from build123d import *

# Parameters (mm, degrees)
BOSS_EXTRUDE1_DEPTH            = 1.93
BOSS_EXTRUDE2_START            = 1.93
BOSS_EXTRUDE2_DEPTH            = 5
BOSS_EXTRUDE3_DEPTH            = 19
CUT_EXTRUDE1_REACH             = 69.337
CUT_EXTRUDE1_DIRECTION_2_REACH = 69.337
FILLET1_R                      = 6
CUT_EXTRUDE2_REACH             = 69.337
SKETCH5_R                      = 3
CUT_EXTRUDE2_DIRECTION_2_REACH = 69.337


with BuildPart() as part:
    # Sketch1 → Boss-Extrude1 (new body)
    # profile 1 of 4: a face of its own
    with BuildSketch(Plane.XY):
        with BuildLine():
            ThreePointArc((32, 27.202941017), (0, 42), (-32, 27.202941017))
            Line((-32, 27.202941017), (-32, 17.202941017))
            Line((-32, 17.202941017), (-37, 11.488655303))
            Line((-37, 11.488655303), (-37, -25.449961479))
            Line((-37, -25.449961479), (-34, -25.449961479))
            Line((-34, -25.449961479), (-34, -26.449961479))
            Line((-34, -26.449961479), (-28, -26.449961479))
            ThreePointArc((-28, -26.449961479), (0, -38.517534478), (28, -26.449961479))
            Line((28, -26.449961479), (34, -26.449961479))
            Line((34, -26.449961479), (34, -25.449961479))
            Line((34, -25.449961479), (37, -25.449961479))
            Line((37, -25.449961479), (37, 11.488655303))
            Line((37, 11.488655303), (32, 17.202941017))
            Line((32, 17.202941017), (32, 27.202941017))
        make_face()
        with BuildLine():
            Line((-13.076696831, -27), (-14, -27))
            ThreePointArc((-14, -27), (-18.345139389, -25.488147565), (-20.813361759, -21.605646769))
            ThreePointArc((-20.813361759, -21.605646769), (0, 30), (20.813361759, -21.605646769))
            ThreePointArc((20.813361759, -21.605646769), (18.345139389, -25.488147565), (14, -27))
            Line((14, -27), (13.076696831, -27))
            ThreePointArc((13.076696831, -27), (0, -30), (-13.076696831, -27))
        make_face(mode=Mode.SUBTRACT)
    # profile 2 of 4: a face of its own
    with BuildSketch(Plane.XY):
        Polygon((-37, -25.449961479), (-37, 11.488655303), (-39, 9.202941017), (-39, -25.449961479), align=None)
    # profile 3 of 4: a face of its own
    with BuildSketch(Plane.XY):
        Polygon((39, 9.202941017), (37, 11.488655303), (37, -25.449961479), (39, -25.449961479), align=None)
    # profile 4 of 4: a face of its own
    with BuildSketch(Plane.XY):
        with BuildLine():
            Line((-28, -26.449961479), (-34, -26.449961479))
            Line((-34, -26.449961479), (-34, -32.449961479))
            ThreePointArc((-34, -32.449961479), (0, -47), (34, -32.449961479))
            Line((34, -32.449961479), (34, -26.449961479))
            Line((34, -26.449961479), (28, -26.449961479))
            ThreePointArc((28, -26.449961479), (0, -38.517534478), (-28, -26.449961479))
        make_face()
    extrude(amount=BOSS_EXTRUDE1_DEPTH)

    # Sketch1<3> → Boss-Extrude2 (add)
    with BuildSketch(Plane.XY.offset(BOSS_EXTRUDE2_START)):
        with BuildLine():
            Line((-27, -43.854874301), (-34, -34.949961479))
            Line((-34, -34.949961479), (-34, -32.449961479))
            ThreePointArc((-34, -32.449961479), (0, -47), (34, -32.449961479))
            Line((34, -32.449961479), (34, -34.949961479))
            Line((34, -34.949961479), (27, -43.854874301))
            ThreePointArc((27, -43.854874301), (0, -51.5), (-27, -43.854874301))
        make_face()
        with BuildLine():
            Line((-28, -26.449961479), (-34, -26.449961479))
            Line((-34, -26.449961479), (-34, -32.449961479))
            ThreePointArc((-34, -32.449961479), (0, -47), (34, -32.449961479))
            Line((34, -32.449961479), (34, -26.449961479))
            Line((34, -26.449961479), (28, -26.449961479))
            ThreePointArc((28, -26.449961479), (0, -38.517534478), (-28, -26.449961479))
        make_face()
    extrude(amount=BOSS_EXTRUDE2_DEPTH)

    # Sketch1<4> → Boss-Extrude3 (add)
    with BuildSketch(Plane.XY):
        Polygon((-37, -25.449961479), (-37, 11.488655303), (-39, 9.202941017), (-39, -25.449961479), align=None)
        Polygon((39, 9.202941017), (37, 11.488655303), (37, -25.449961479), (39, -25.449961479), align=None)
    extrude(amount=BOSS_EXTRUDE3_DEPTH)

    # Sketch3 → Cut-Extrude1 (cut, up to next)
    with BuildSketch(Plane(origin=(0, 0, 0), x_dir=(0, 0, -1), z_dir=(1, 0, 0)), mode=Mode.PRIVATE) as cut_extrude1_sk1:
        Polygon((-1.93, 11.488655303), (-19, -10.449961479), (-19, 9.202941017), (-19, 11.488655303), align=None)
    cut_extrude1_tool1 = extrude(cut_extrude1_sk1.sketch, amount=-CUT_EXTRUDE1_REACH, mode=Mode.PRIVATE) & part.part
    add(cut_extrude1_tool1.solids().sort_by_distance((0, 4.175783, 13.31))[0], mode=Mode.SUBTRACT)

    # Sketch3 → Cut-Extrude1 direction 2 (cut, up to next)
    with BuildSketch(Plane(origin=(0, 0, 0), x_dir=(0, 0, -1), z_dir=(1, 0, 0)), mode=Mode.PRIVATE) as cut_extrude1_direction_2_sk1:
        Polygon((-1.93, 11.488655303), (-19, -10.449961479), (-19, 9.202941017), (-19, 11.488655303), align=None)
    cut_extrude1_direction_2_tool1 = extrude(cut_extrude1_direction_2_sk1.sketch, amount=CUT_EXTRUDE1_DIRECTION_2_REACH, mode=Mode.PRIVATE) & part.part
    add(cut_extrude1_direction_2_tool1.solids().sort_by_distance((0, 4.175783, 13.31))[0], mode=Mode.SUBTRACT)

    # Fillet1
    fillet1_edges = [part.edges().sort_by_distance(p)[0] for p in [
        (38, -25.449961479, 19),
        (38, -10.449961479, 19),
        (-38, -10.449961479, 19),
        (-38, -25.449961479, 19),
    ]]
    fillet(fillet1_edges, radius=FILLET1_R)

    # Sketch5 → Cut-Extrude2 (cut, up to next)
    with BuildSketch(Plane(origin=(0, 0, 0), x_dir=(0, 0, -1), z_dir=(1, 0, 0)), mode=Mode.PRIVATE) as cut_extrude2_sk1:
        with Locations(Location((-13, -19.449961479, 0), (0, 0, 180))):
            Circle(SKETCH5_R)
    cut_extrude2_tool1 = extrude(cut_extrude2_sk1.sketch, amount=-CUT_EXTRUDE2_REACH, mode=Mode.PRIVATE) & part.part
    add(cut_extrude2_tool1.solids().sort_by_distance((0, -19.449961, 13))[0], mode=Mode.SUBTRACT)

    # Sketch5 → Cut-Extrude2 direction 2 (cut, up to next)
    with BuildSketch(Plane(origin=(0, 0, 0), x_dir=(0, 0, -1), z_dir=(1, 0, 0)), mode=Mode.PRIVATE) as cut_extrude2_direction_2_sk1:
        with Locations(Location((-13, -19.449961479, 0), (0, 0, 180))):
            Circle(SKETCH5_R)
    cut_extrude2_direction_2_tool1 = extrude(cut_extrude2_direction_2_sk1.sketch, amount=CUT_EXTRUDE2_DIRECTION_2_REACH, mode=Mode.PRIVATE) & part.part
    add(cut_extrude2_direction_2_tool1.solids().sort_by_distance((0, -19.449961, 13))[0], mode=Mode.SUBTRACT)


solid = part.part
Input: part model. Units: mm. Frame: model coordinates. A direction names the side the tool comes from. Coordinates: 2 decimals unless noted, no trailing zeros. Order: outer loops, then holes, each group sorted by start corner. A loop starts at its lowest first (then second) coordinate and runs counter-clockwise, first axis right, second up. Notation, with made-up numbers: M 28,65.5 L 86,65.5 A29 cw 86,89.5 Z; hole C 80.25,2 d8. An arc over 180 degrees is marked long. Answer in a Markdown table with one row per item.
(1) Section query A-A, the plane x = 0. Output: boundary loops of the cut face in (y, z), plus the area to 3 significant figures.
Numbers:
| item | result |
|---|---|
| outline | M -51.5,1.93 L -47,1.93 L -47,0 L -30,0 L -30,1.93 L -38.52,1.93 L -38.52,6.93 L -51.5,6.93 Z; M 30,0 L 42,0 L 42,1.93 L 30,1.93 Z |
| area | 121 mm^2 |
(2) Material intervals for line 1 (X direction, y = -4, z = 7.5); line 2 (X direction, y = 0, z = 0.9); line 3 (Z direction, x = -25, y = -35.5), sorted ascending. Write a range as [from, to].
Numbers:
| item | result |
|---|---|
| line 1 | x = [-39, -37], [37, 39] |
| line 2 | x = [-39, -30], [30, 39] |
| line 3 | z = [0, 6.93] |
(3) Access query for faces 1 (the flat face through (0, -48, 1.93)), 2 (the flat face through (32, 22, 1)), 3 (the flat face through (-38, -25.45, 6)). Directions: +Z, -Z, +X, -X, +Y, -Y. A direction counts if a zero-diameter tool reaches every point of the face in a straight line with its end or side. Return the directions, or none.
Numbers:
| item | result |
|---|---|
| face 1 | -Z, -Y |
| face 2 | +Z, -Z, +X, +Y |
| face 3 | +Z, -Z, -X, -Y |
(4) Section query C-C, the plane y = 26. Output: boundary loops of the cut face in (x, z), plus the area to 3 significant figures.
Numbers:
| item | result |
|---|---|
| outline | M -32,0 L -14.97,0 L -14.97,1.93 L -32,1.93 Z; M 14.97,0 L 32,0 L 32,1.93 L 14.97,1.93 Z |
| area | 65.7 mm^2 |
(5) Section query B-B, the plane z = 5. Output: boundary loops of the cut face in (x, y), plus the area to 3 significant figures.
Numbers:
| item | result |
|---|---|
| outline | M -39,-25.45 L -37,-25.45 L -37,7.54 L -39,7.54 Z; M -34,-34.95 L -27,-43.85 A51.5 ccw 27,-43.85 L 34,-34.95 L 34,-26.45 L 28,-26.45 A38.52 cw -28,-26.45 L -34,-26.45 Z; M 37,-25.45 L 39,-25.45 L 39,7.54 L 37,7.54 Z |
| area | 1,070 mm^2 |
(6) Contact query for flat-ended pins moving along their axis: pin 1 Ø10 at (x, y) = (-12, 25.5) entering from +Z; pin 2 Ø2.5 at (x, z) = (-37, 8) entering from -Y; pin 3 Ø5.5 at (x, z) = (35.5, 8) entering from -Y. Output: stop coordinate, or through.
Numbers:
| item | result |
|---|---|
| pin 1 | stops at z = 1.93 |
| pin 2 | stops at y = -25.45 |
| pin 3 | stops at y = -36.26 |
(7) Section query D-D, the plane y = -18. Output: boundary loops of the cut face in (x, z), plus the area to 3 significant figures.
Numbers:
| item | result |
|---|---|
| outline | M -39,0 L -24,0 L -24,1.93 L -37,1.93 L -37,10.37 L -39,10.37 Z; M -39,15.63 L -37,15.63 L -37,19 L -39,19 Z; M 24,0 L 39,0 L 39,10.37 L 37,10.37 L 37,1.93 L 24,1.93 Z; M 37,15.63 L 39,15.63 L 39,19 L 37,19 Z |
| area | 105 mm^2 |
(8) Draft query along X for faces 4 (the flat face through (-30.451, -39.465, 4.395)), 5 (the flat face through (34, -30, 3)), 6 (the flat face through (0, -39, 6.93)), 7 (the cylindrical face through (0.439, -38.515, 4.395)). Return one class per face: pulls with the +X half, pulls with the -X half, needs draft (parallel to the pull), parting line crosses it, or undercut.
Numbers:
| item | result |
|---|---|
| face 4 | pulls with the -X half |
| face 5 | pulls with the +X half |
| face 6 | needs draft |
| face 7 | undercut |
